```python
from build123d import *

# Parameters (mm, degrees)
ESQUISSE1_R        = 53.5
ESQUISSE1_R_2      = 1
ESQUISSE1_R_3      = 3
BOSS_EXTRU_1_DEPTH = 1.6


with BuildPart() as part:
    # Esquisse1 → Boss.-Extru.1 (new body)
    with BuildSketch(Plane.XY):
        Circle(ESQUISSE1_R)
        with Locations((35, 0)):
            Circle(ESQUISSE1_R_2, mode=Mode.SUBTRACT)
        with Locations((17.5, -30.310889132)):
            Circle(ESQUISSE1_R_2, mode=Mode.SUBTRACT)
        with Locations((-17.5, -30.310889132)):
            Circle(ESQUISSE1_R_2, mode=Mode.SUBTRACT)
        with Locations((-35, 0)):
            Circle(ESQUISSE1_R_2, mode=Mode.SUBTRACT)
        with Locations((-17.5, 30.310889132)):
            Circle(ESQUISSE1_R_2, mode=Mode.SUBTRACT)
        with Locations((17.5, 30.310889132)):
            Circle(ESQUISSE1_R_2, mode=Mode.SUBTRACT)
        with Locations((0, -15)):
            Circle(ESQUISSE1_R_3, mode=Mode.SUBTRACT)
        with Locations((12.990381057, -7.5)):
            Circle(ESQUISSE1_R_3, mode=Mode.SUBTRACT)
        with Locations((12.990381057, 7.5)):
            Circle(ESQUISSE1_R_3, mode=Mode.SUBTRACT)
        with Locations((0, 15)):
            Circle(ESQUISSE1_R_3, mode=Mode.SUBTRACT)
        with Locations((-12.990381057, 7.5)):
            Circle(ESQUISSE1_R_3, mode=Mode.SUBTRACT)
    extrude(amount=BOSS_EXTRU_1_DEPTH)


solid = part.part
```
The model under review builds one solid part; all positions refer to its coordinate system, in mm. Round coordinates to 2 decimals unless told otherwise and drop trailing zeros. Write each loop counter-clockwise with the first axis right and the second up, starting at its lowest first coordinate (ties: lowest second). Pieces come first, ordered by that corner, then holes.
(1) We need section D-D on x = 14. Give the boundary of the cut face in (y, z) (3 decimals), and give its area (3 significant figures).
(2) Wall thickness on L1, parallel to Y at x = 0, z = 1.2; L2, parallel to Y at x = -1, z = 1.05; L3, parallel to X at y = 31, z = 1.3: over which ranges is each line inside the solid? List them lowest first.
(3) Insertion check: pin 1 (5 mm diameter, centred on x = 22, y = -2, fed in from -Z); pin 2 (1.2 mm diameter, centred on x = 17.5, y = 30.31, fed in from +Z). Each pin has a flat end and moves straight along its axis. Give the tip position at first contact, or say it passes through.
(4) We need section C-C on z = 0.9. Give the number of separate pieces and of enclosed holes in the cut face, and give its area (3 significant figures).
(5) We need section A-A on x = 0. Give the boundary of the cut face in (y, z).
(6) We need section B-B on y = 15. Give the boundary of the cut face in (x, z).
Findings below:
1. outline: (-51.636, 0) - (-10.325, 0) - (-10.325, 1.6) - (-51.636, 1.6) - close; (-4.675, 0) - (4.675, 0) - (4.675, 1.6) - (-4.675, 1.6) - close; (10.325, 0) - (51.636, 0) - (51.636, 1.6) - (10.325, 1.6) - close
1. area: 147 mm2
2. L1: y = -53.5 to -18, -12 to 12, 18 to 53.5
2. L2: y = -53.49 to -17.83, -12.17 to 12.17, 17.83 to 53.49
2. L3: x = -43.6 to -18.22, -16.78 to 16.78, 18.22 to 43.6
3. pin 1: stops at z = 0
3. pin 2: passes through
4. separate pieces: 1
4. enclosed holes: 11
4. area: 8,830 mm2
5. outline: (-53.5, 0) - (-18, 0) - (-18, 1.6) - (-53.5, 1.6) - close; (-12, 0) - (12, 0) - (12, 1.6) - (-12, 1.6) - close; (18, 0) - (53.5, 0) - (53.5, 1.6) - (18, 1.6) - close
6. outline: (-51.35, 0) - (-3, 0) - (-3, 1.6) - (-51.35, 1.6) - close; (3, 0) - (51.35, 0) - (51.35, 1.6) - (3, 1.6) - close
